Check sheet for the modelled part. Datum: model origin and axes. Units: mm. Round coordinates to 2 decimals unless told otherwise and drop trailing zeros. Write each loop counter-clockwise with the first axis right and the second up, starting at its lowest first coordinate (ties: lowest second). Pieces come first, ordered by that corner, then holes.
Item 1: Cross-section at C-C on x = -22. Enter the section's corners in (y, z), plus the area to 3 significant figures.
Item 2: Cross-section at B-B on y = 14.5. Enter the section's corners in (x, z), plus the area to 3 significant figures.
Item 3: Cross-section at A-A on z = 26.5. Enter the section's corners in (x, y), plus the area to 3 significant figures.
Item 4: Material ranges on line 1 (X direction, y = 6, z = 37); line 2 (X direction, y = 26, z = 6); line 3 (Y direction, x = -6.5, z = 7), recorded low to high.
Item 5: Go/stop test with flat-tipped pins: pin 1 Ø12 at (x, z) = (-24, 18) entering from -Y; pin 2 Ø10 at (x, z) = (-12.5, 19) entering from -Y; pin 3 Ø2 at (x, z) = (-16.5, 18) entering from -Y. Record where each tip stops, or that it passes through.
from build123d import *

# Parameters (mm, degrees)
EXTRUDE_1_DEPTH = 40


with BuildPart() as part:
    # 草图1 → 凸台-拉伸1 (new body)
    with BuildSketch(Plane.XY):
        with BuildLine():
            Line((-8.460821473, -7.099472177), (-27.703402524, 15.832942921))
            ThreePointArc((-27.703402524, 15.832942921), (-29.252585633, 27.600156893), (-19.242581051, 33.977233123))
            Line((-19.242581051, 33.977233123), (11.044818024, 33.977233123))
            Line((11.044818024, 33.977233123), (11.044818024, 0))
            ThreePointArc((11.044818024, 0), (3.777550244, -10.378733995), (-8.460821473, -7.099472177))
        make_face()
    extrude(amount=EXTRUDE_1_DEPTH)


solid = part.part
Response values:
1. outline: (9.04, 0) - (33.63, 0) - (33.63, 40) - (9.04, 40) - close
1. area: 984 mm2
2. outline: (-26.58, 0) - (11.04, 0) - (11.04, 40) - (-26.58, 40) - close
2. area: 1,510 mm2
3. outline: (-27.7, 15.83) - (-8.46, -7.1) arc R11.04 ccw to (11.04, 0) - (11.04, 33.98) - (-19.24, 33.98) arc R11.04 ccw to start
3. area: 1,430 mm2
4. line 1: x = -19.45 to 11.04
4. line 2: x = -29.85 to 11.04
4. line 3: y = -8.93 to 33.98
5. pin 1: stops at y = 4.27
5. pin 2: stops at y = -8.11
5. pin 3: stops at y = 1.29
